Build history of the part. All positions in model axes, mm. Coordinates: 2 decimals unless noted, no trailing zeros. Loops run counter-clockwise (first coordinate to the right, second up) from the corner with the lowest first, then second, coordinate; pieces in that order, holes last. Notation, with made-up numbers: (-39.75, -29.5) - (-6.75, -29.5) arc R25 ccw to (-6.75, -9.5) - close; hole circle Ø4 at (31, -36.5). An arc over 180 degrees is marked (long way). One line per item, written item: value.
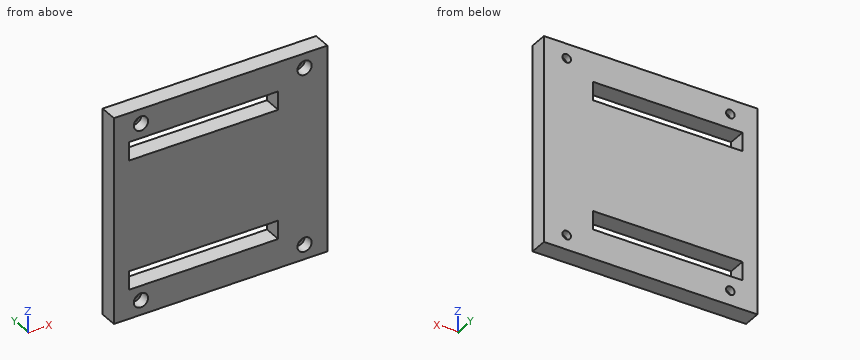
```python
from build123d import *

# Parameters (mm, degrees)
SKETCH_1_W          = 30
SKETCH_1_H          = 29
SKETCH_1_W_2        = 21
SKETCH_1_H_2        = 2.6
EXTRUDE_1_DEPTH     = 2.5
SKETCH_2_R          = 0.6
CUT_EXTRUDE_1_DEPTH = 22.011901389
SKETCH_2_3_R        = 1
SKETCH_2_3_R_2      = 0.6
CUT_EXTRUDE_2_DEPTH = 1.5


with BuildPart() as part:
    # Sketch 1 → Extrude 1 (new body)
    with BuildSketch(Plane(origin=(0, 0, 0), x_dir=(1, 0, 0), z_dir=(0, 1, 0))):
        Rectangle(SKETCH_1_W, SKETCH_1_H)
        with Locations((-2.4, 9.1)):
            Rectangle(SKETCH_1_W_2, SKETCH_1_H_2, mode=Mode.SUBTRACT)
        with Locations((-2.4, -9.1)):
            Rectangle(SKETCH_1_W_2, SKETCH_1_H_2, mode=Mode.SUBTRACT)
    extrude(amount=EXTRUDE_1_DEPTH)

    # Sketch 2 → Cut-Extrude 1 (cut, through all)
    with BuildSketch(Plane.XZ):
        with Locations(Location((-11.2, -12.45, 0), (0, 0, 270))):
            Circle(SKETCH_2_R)
        with Locations(Location((-11.2, 12.45, 0), (0, 0, 270))):
            Circle(SKETCH_2_R)
        with Locations(Location((11.8, 12.45, 0), (0, 0, 270))):
            Circle(SKETCH_2_R)
        with Locations(Location((11.8, -12.45, 0), (0, 0, 270))):
            Circle(SKETCH_2_R)
    extrude(amount=-CUT_EXTRUDE_1_DEPTH, mode=Mode.SUBTRACT)

    # Sketch 2_3 → Cut-Extrude 2 (cut)
    # profile 1 of 4: a face of its own
    with BuildSketch(Plane.XZ):
        with Locations(Location((-11.2, -12.45, 0), (0, 0, 270))):
            Circle(SKETCH_2_3_R)
        with Locations(Location((-11.2, -12.45, 0), (0, 0, 270))):
            Circle(SKETCH_2_3_R_2, mode=Mode.SUBTRACT)
    # profile 2 of 4: a face of its own
    with BuildSketch(Plane.XZ):
        with Locations(Location((-11.2, 12.45, 0), (0, 0, 270))):
            Circle(SKETCH_2_3_R)
        with Locations(Location((-11.2, 12.45, 0), (0, 0, 270))):
            Circle(SKETCH_2_3_R_2, mode=Mode.SUBTRACT)
    # profile 3 of 4: a face of its own
    with BuildSketch(Plane.XZ):
        with Locations(Location((11.8, 12.45, 0), (0, 0, 270))):
            Circle(SKETCH_2_3_R)
        with Locations(Location((11.8, 12.45, 0), (0, 0, 270))):
            Circle(SKETCH_2_3_R_2, mode=Mode.SUBTRACT)
    # profile 4 of 4: a face of its own
    with BuildSketch(Plane.XZ):
        with Locations(Location((11.8, -12.45, 0), (0, 0, 270))):
            Circle(SKETCH_2_3_R)
        with Locations(Location((11.8, -12.45, 0), (0, 0, 270))):
            Circle(SKETCH_2_3_R_2, mode=Mode.SUBTRACT)
    extrude(amount=-CUT_EXTRUDE_2_DEPTH, mode=Mode.SUBTRACT)


solid = part.part
```
Item 1: Cut at A-A, the plane x = -7.5. Write the cut outline in (y, z), then the cut area to 3 significant figures.
Check result:
outline: (0, -14.5) - (2.5, -14.5) - (2.5, -10.4) - (0, -10.4) - close; (0, -7.8) - (2.5, -7.8) - (2.5, 7.8) - (0, 7.8) - close; (0, 10.4) - (2.5, 10.4) - (2.5, 14.5) - (0, 14.5) - close
area: 59.5 mm^2
Item 2: Drop a flat-ended pin along its axis: P1, Ø1.4, axis at x = -11.2, z = -12.45, coming from the -Y side. Give the stop position or say it passes through.
Check result:
P1: stops at y = 1.5
Item 3: Cut at D-D, the plane x = -11.2. Write the cut outline in (y, z), then the cut area to 3 significant figures.
Check result:
outline: (0, -14.5) - (2.5, -14.5) - (2.5, -13.05) - (1.5, -13.05) - (1.5, -13.45) - (0, -13.45) - close; (0, -11.45) - (1.5, -11.45) - (1.5, -11.85) - (2.5, -11.85) - (2.5, -10.4) - (0, -10.4) - close; (0, -7.8) - (2.5, -7.8) - (2.5, 7.8) - (0, 7.8) - close; (0, 10.4) - (2.5, 10.4) - (2.5, 11.85) - (1.5, 11.85) - (1.5, 11.45) - (0, 11.45) - close; (0, 13.45) - (1.5, 13.45) - (1.5, 13.05) - (2.5, 13.05) - (2.5, 14.5) - (0, 14.5) - close
area: 51.1 mm^2
Item 4: Cut at B-B, the plane z = -12.45. Write the cut outline in (x, y), then the cut area to 3 significant figures.
Check result:
outline: (-15, 0) - (-12.2, 0) - (-12.2, 1.5) - (-11.8, 1.5) - (-11.8, 2.5) - (-15, 2.5) - close; (-10.6, 1.5) - (-10.2, 1.5) - (-10.2, 0) - (10.8, 0) - (10.8, 1.5) - (11.2, 1.5) - (11.2, 2.5) - (-10.6, 2.5) - close; (12.4, 1.5) - (12.8, 1.5) - (12.8, 0) - (15, 0) - (15, 2.5) - (12.4, 2.5) - close
area: 66.6 mm^2
Item 5: Cut at C-C, the plane y = 2.15. Write the cut outline in (x, z).
Check result:
outline: (-15, -14.5) - (15, -14.5) - (15, 14.5) - (-15, 14.5) - close; hole (-12.9, -10.4) - (8.1, -10.4) - (8.1, -7.8) - (-12.9, -7.8) - close; hole (-12.9, 7.8) - (8.1, 7.8) - (8.1, 10.4) - (-12.9, 10.4) - close; hole circle Ø1.2 at (-11.2, -12.45); hole circle Ø1.2 at (-11.2, 12.45); hole circle Ø1.2 at (11.8, -12.45); hole circle Ø1.2 at (11.8, 12.45)
Item 6: Probe probe 1 along X at (y, z) = (0.55, 12.45); probe 2 along X at (y, z) = (1.95, 12.45); probe 3 along Z at (x, y) = (-1.5, 1.45). List the from-to ranges inside material, lowest first. Write a range as from..to.
Check result:
probe 1: x = -15..-12.2, -10.2..10.8, 12.8..15
probe 2: x = -15..-11.8, -10.6..11.2, 12.4..15
probe 3: z = -14.5..-10.4, -7.8..7.8, 10.4..14.5
